from build123d import *

# Parameters (mm, degrees)
SKETCH8_R             = 1.825
M4X0_7_TAPPED_HOLE1_D = 3.3
CIRPATTERN1_COUNT     = 8


with BuildPart() as part:
    # Sketch3 → Revolve1 (revolve)
    with BuildSketch(Plane.XY, mode=Mode.PRIVATE) as revolve1_sk:
        Polygon((86.2847, 16.644516882), (86.2847, 0), (76.2847, 0), (76.2847, 16.644516882), (78.5347, 25.041631199), (84.0347, 25.041631199), align=None)
    revolve(revolve1_sk.sketch.rotate(Axis((0, 0, 0), (0, 1, 0)), 90), axis=Axis((0, 0, 0), (0, 1, 0)))

    # Sketch8 → Cut-Revolve1 (revolve, cut)
    with BuildSketch(Plane.XY, mode=Mode.PRIVATE) as cut_revolve1_sk:
        with Locations((81.2847, 25.041631199)):
            Circle(SKETCH8_R)
    revolve(cut_revolve1_sk.sketch.rotate(Axis((0, 0, 0), (0, 1, 0)), 90), axis=Axis((0, 0, 0), (0, 1, 0)), mode=Mode.SUBTRACT)

    # Sketch15 → Cut-Revolve3 (revolve, cut)
    with BuildSketch(Plane.XY, mode=Mode.PRIVATE) as cut_revolve3_sk:
        Polygon((81.2847, 25.041631199), (78.5347, 25.041631199), (78.266750808, 24.041631199), (81.2847, 24.041631199), align=None)
    revolve(cut_revolve3_sk.sketch.rotate(Axis((0, 0, 0), (0, 1, 0)), 90), axis=Axis((0, 0, 0), (0, 1, 0)), mode=Mode.SUBTRACT)

    # Sketch17 → Revolve3 (revolve)
    with BuildSketch(Plane.XY, mode=Mode.PRIVATE) as revolve3_sk:
        Polygon((84.1097, 27.041631199), (83.1097, 27.041631199), (83.1097, 25.041631199), (84.0347, 25.041631199), (86.2847, 16.644516882), align=None)
    revolve(revolve3_sk.sketch.rotate(Axis((0, 0, 0), (0, 1, 0)), 90), axis=Axis((0, 0, 0), (0, 1, 0)))

    # M4x0.7 Tapped Hole1 (through all)
    with Locations(Plane(origin=(0, 0, 0), x_dir=(-1, 0, 0), z_dir=(0, -1, 0))):
        with Locations((0, -81)):
            m4x0_7_tapped_hole1 = Hole(M4X0_7_TAPPED_HOLE1_D / 2)

    # CirPattern1: M4x0.7 Tapped Hole1 ×8 about axis
    cirpattern1_axis = Axis((0, 0, 0), (0, 1, 0))
    for i in range(1, CIRPATTERN1_COUNT):
        add(m4x0_7_tapped_hole1.rotate(cirpattern1_axis, i * 360 / CIRPATTERN1_COUNT), mode=Mode.SUBTRACT)


solid = part.part
Can you work these out from the model? Positions are in its coordinate system, mm. A direction names the side the tool comes from. Coordinates: 2 decimals unless noted, no trailing zeros. Write each question's results on one line, items separated by ' | '. Start each with the question number.
Item 1: Thinking about a two-plate mould opening in Z: for faces 3 (the flat face through (76.3, 0, -6)), 4 (the cylindrical face through (33.048, 8.206, -79.705)), 5 (the flat face through (53, 24.042, 59)), which applies, released by +Z, released by -Z, zero draft, split by the parting line, or undercut?
Item 2: On a 3-axis mill with a long thin cutter (end or side, diameter ignored), from which of +Z, -Z, +X, -X, +Y, -Y can I reach the whole of each face in a straight line? I mean faces 1 (the cylindrical face through (50.571, 26.028, 65.953)), 2 (the cylindrical face through (-22.914, 8.439, -72.762)). Say none if no direction works.
Item 3: I'm going to push flat-ended pins straight in: P1, Ø1, axis at y = 21.5, z = 0.5, coming from the -X side; P2, Ø2, axis at x = 38.5, y = 15.5, coming from the +Z side; P3, Ø1.5, axis at y = 13.5, z = 13.5, coming from the +X side. Where does each tip first touch, or does it pass through?
Item 4: Please list where these lines run through material, in increasing order: probe 1 along Z at (x, y) = (-0.5, 19.25); probe 2 along X at (y, z) = (18.5, 31.5); probe 3 along X at (y, z) = (26, -71.5).
Item 5: If we section it at A-A, the plane y = 19.25: Count the separate pieces of the cut face and the enclosed holes in it, and give its area (3 significant figures).
Answer block:
1) face 3: zero draft | face 4: split by the parting line | face 5: undercut
2) face 1: +Y | face 2: +Y, -Y
3) P1: x = -85.37 | P2: z = 77.71 | P3: x = 85.34
4) probe 1: -85.74 to -82.57, -79.43 to -76.98, 76.98 to 79.43, 82.57 to 85.74 | probe 2: -79.91 to -70.02, 70.02 to 79.91 | probe 3: -44.71 to -42.37, 42.37 to 44.71
5) separate pieces: 1 | enclosed holes: 9 | area: 4,410 mm²
